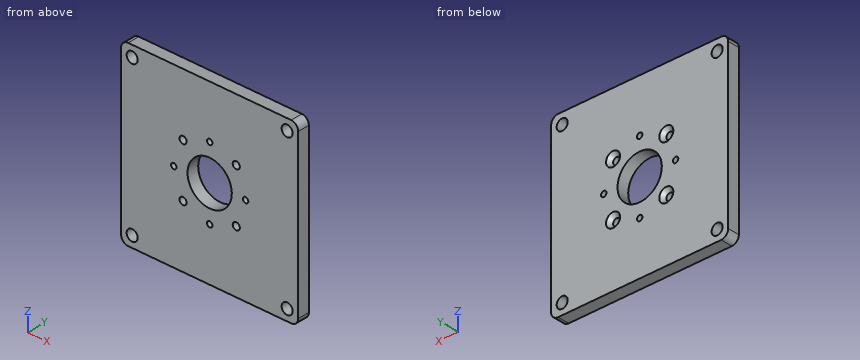
Autodesk Inventor part; units mm, degrees
ref_plane "YZ Plane" through (0, 0, 0) normal (1, 0, 0) x (0, 1, 0)
ref_plane "XZ Plane" through (0, 0, 0) normal (0, 1, 0) x (-1, 0, 0)
ref_plane "XY Plane" through (0, 0, 0) normal (0, 0, 1) x (1, 0, 0)
sketch "Sketch1" plane through (0, 0, 0) normal (0, 1, 0) x (-1, 0, 0)
  line L0 (40, 36.825) -> (40, -36.825)
  line L1 (36.825, -40) -> (-36.825, -40)
  line L2 (-40, -36.825) -> (-40, 36.825)
  line L3 (-36.825, 40) -> (-13.175, 40)
  line L4 (13.175, 40) -> (36.825, 40)
  arc A0 (40, 36.825) -> (36.825, 40) centre (36.825, 36.825) ccw
  arc A1 (36.825, -40) -> (40, -36.825) centre (36.825, -36.825) ccw
  arc A2 (-40, -36.825) -> (-36.825, -40) centre (-36.825, -36.825) ccw
  arc A3 (-36.825, 40) -> (-40, 36.825) centre (-36.825, 36.825) ccw
  line L5 (13.175, 40) -> (-13.175, 40)
  point P0 (0, 0)
  point P1 (40, 40)
  point P2 (40, -40)
  point P3 (-40, -40)
  point P4 (-40, 40)
  point P5 (-10, 40)
  point P6 (10, 40)
  point P7 (40, 0)
  point P8 (0, -40)
  point P9 (0, 60)
  dimension "d0" = 80
  dimension "d1" = 80
  dimension "d27" = 3.175
extrude "Extrusion1" add sketch "Sketch1" along normal blind 5.334
sketch "Sketch2" plane through (0, 5.334, 0) normal (0, 1, 0) x (1, 0, 0)
  line L0 (-12.0208, -12.0208) -> (0, 0)
  line L1 (0, 0) -> (-40, 0)
  line L2 (-40, 36.825) -> (-40, -36.825)
  point P0 (-17.5, 17.5)
  point P1 (-17.5, -17.5)
  point P2 (12.0208, -12.0208)
  point P3 (12.0208, 12.0208)
  point P4 (-12.0208, 12.0208)
  dimension "d6" = 17
  dimension "d7" = 45
  dimension "d10" = 360
hole "Hole1" at (-12.0208, 5.334, 12.0208) at (12.0208, 5.334, 12.0208) at (12.0208, 5.334, -12.0208) at (-12.0208, 5.334, -12.0208) direction (0, -1, 0) diameter 3.2 end through all countersink diameter 6.35 countersink angle 82
sketch "Sketch3" plane through (0, 5.334, 0) normal (0, 1, 0) x (1, 0, 0)
  point P0 (0, 0)
  point P1 (0, 0)
hole "Hole2" at (0, 5.334, 0) direction (0, -1, 0) diameter 20 end through all
sketch "Sketch4" plane through (0, 5.334, 0) normal (0, 1, 0) x (1, 0, 0)
  point P0 (0, 0)
  point P1 (-16.215, 0)
  point P2 (0, -16.215)
  point P3 (16.215, 0)
  point P4 (0, 16.215)
  dimension "d29" = 16.215
  dimension "d47" = 360
hole "Hole3" at (-16.215, 5.334, 0) at (0, 5.334, 16.215) at (16.215, 5.334, 0) at (0, 5.334, -16.215) direction (0, -1, 0) diameter 2.4638 end through all
sketch "Sketch7" plane through (0, 5.334, 0) normal (0, 1, 0) x (1, 0, 0)
  line L0 (-40, 36.825) -> (-40, -36.825)
  line L1 (36.825, 40) -> (-36.825, 40)
  line L2 (-36.825, -40) -> (36.825, -40)
  line L3 (40, -36.825) -> (40, 36.825)
  point P0 (0, 0)
  point P1 (-35, 35)
  point P2 (35, 35)
  point P3 (35, -35)
  point P4 (-35, -35)
  dimension "d49" = 5
  dimension "d50" = 5
  dimension "d51" = 5
  dimension "d52" = 5
hole "Hole4" at (-35, 5.334, -35) at (35, 5.334, -35) at (35, 5.334, 35) at (-35, 5.334, 35) direction (0, -1, 0) diameter 5 end through all
properties part number "base_mount"
Model file for the job. Use its own axes, mm. Give positions to 0.01 mm unless a question says otherwise; leave off trailing zeros. Loops run counter-clockwise (first coordinate to the right, second up) from the corner with the lowest first, then second, coordinate; pieces in that order, holes last.
1) Saw through at C-C (z = -35). Write the cut outline in (x, y), plus the area to 3 significant figures.
2) Saw through at D-D (y = 1.2). Count the separate pieces of the cut face and the enclosed holes in it, plus the area to 3 significant figures.
3) Saw through at A-A (z = 0). Write the cut outline in (x, y).
4) Saw through at B-B (x = 0). Write the cut outline in (y, z), plus the area to 3 significant figures.
5) Wall check: line 1 (X direction, y = 3.4, z = -35); line 2 (Z direction, x = -33, y = 5); line 3 (X direction, y = 3.4, z = 12). Give the ranges that are in metal, low to high.
Answer block:
1. outline: (-40, 0) - (-37.5, 0) - (-37.5, 5.33) - (-40, 5.33) - close; (-32.5, 0) - (32.5, 0) - (32.5, 5.33) - (-32.5, 5.33) - close; (37.5, 0) - (40, 0) - (40, 5.33) - (37.5, 5.33) - close
1. area: 373 mm2
2. separate pieces: 1
2. enclosed holes: 13
2. area: 5,950 mm2
3. outline: (-40, 0) - (-17.45, 0) - (-17.45, 5.33) - (-40, 5.33) - close; (-14.98, 0) - (-10, 0) - (-10, 5.33) - (-14.98, 5.33) - close; (10, 0) - (14.98, 0) - (14.98, 5.33) - (10, 5.33) - close; (17.45, 0) - (40, 0) - (40, 5.33) - (17.45, 5.33) - close
4. outline: (0, -40) - (5.33, -40) - (5.33, -17.45) - (0, -17.45) - close; (0, -14.98) - (5.33, -14.98) - (5.33, -10) - (0, -10) - close; (0, 10) - (5.33, 10) - (5.33, 14.98) - (0, 14.98) - close; (0, 17.45) - (5.33, 17.45) - (5.33, 40) - (0, 40) - close
4. area: 294 mm2
5. line 1: x = -40 to -37.5, -32.5 to 32.5, 37.5 to 40
5. line 2: z = -40 to -36.5, -33.5 to 33.5, 36.5 to 40
5. line 3: x = -40 to -13.62, -10.42 to 10.42, 13.62 to 40
